```python
from build123d import *

# Parameters (mm, degrees)
SKETCH_1_R           = 2.75
SKETCH_1_R_2         = 13
EXTRUDE_1_DEPTH      = 10
EXTRUDE_1_DEPTH_BACK = 10
CUT_EXTRUDE_START    = 7.5
SKETCH_2_R           = 3.3
CUT_EXTRUDE_1_DEPTH  = 33.5
SKETCH_3_R           = 5.4
CUT_EXTRUDE_2_DEPTH  = 1.5
EXTRUDE_START        = 5.95
SKETCH_4_R           = 13
SKETCH_4_R_2         = 5
EXTRUDE_2_DEPTH      = 4
EXTRUDE_2_DEPTH_BACK = 4


with BuildPart() as part:
    # Sketch 1 → Extrude 1 (new body, two sides)
    with BuildSketch(Plane.XY) as extrude_1_sk:
        Polygon((-30, -25), (-30, 7), (-29.5, 7.5), (-17, 7.5), (-17, 17), (-16, 18), (16, 18), (17, 17), (17, 7.5), (29.5, 7.5), (30, 7), (30, -25), align=None)
        with Locations((-23, 0)):
            Circle(SKETCH_1_R, mode=Mode.SUBTRACT)
        with Locations((-23, -18)):
            Circle(SKETCH_1_R, mode=Mode.SUBTRACT)
        with Locations((23, -18)):
            Circle(SKETCH_1_R, mode=Mode.SUBTRACT)
        with Locations((23, 0)):
            Circle(SKETCH_1_R, mode=Mode.SUBTRACT)
        Circle(SKETCH_1_R_2, mode=Mode.SUBTRACT)
    extrude(amount=EXTRUDE_1_DEPTH)
    extrude(extrude_1_sk.sketch, amount=-EXTRUDE_1_DEPTH_BACK)

    # Sketch 2 → Cut-Extrude 1 (cut, through all)
    with BuildSketch(Plane(origin=(0, 0, 0), x_dir=(1, 0, 0), z_dir=(0, 1, 0)).offset(CUT_EXTRUDE_START)):
        with Locations((-23, 0)):
            Circle(SKETCH_2_R)
        with Locations((23, 0)):
            Circle(SKETCH_2_R)
    extrude(amount=-CUT_EXTRUDE_1_DEPTH, mode=Mode.SUBTRACT)

    # Sketch 3 → Cut-Extrude 2 (cut)
    with BuildSketch(Plane(origin=(0, 0, 0), x_dir=(1, 0, 0), z_dir=(0, 1, 0)).offset(CUT_EXTRUDE_START)):
        with Locations((-23, 0)):
            Circle(SKETCH_3_R)
        with Locations((23, 0)):
            Circle(SKETCH_3_R)
    extrude(amount=-CUT_EXTRUDE_2_DEPTH, mode=Mode.SUBTRACT)

    # Sketch 4 → Extrude 2 (add, two sides)
    with BuildSketch(Plane.XY.offset(EXTRUDE_START)) as extrude_2_sk:
        Circle(SKETCH_4_R)
        Circle(SKETCH_4_R_2, mode=Mode.SUBTRACT)
    extrude(amount=EXTRUDE_2_DEPTH)
    extrude(extrude_2_sk.sketch, amount=-EXTRUDE_2_DEPTH_BACK)


solid = part.part
```
Input: part model. Units: mm. Frame: model coordinates. A direction names the side the tool comes from. Round coordinates to 2 decimals unless told otherwise and drop trailing zeros. Order: outer loops, then holes, each group sorted by start corner. A loop starts at its lowest first (then second) coordinate and runs counter-clockwise, first axis right, second up. Notation, with made-up numbers: (-25.75, -9) - (9.25, -9) arc R18 ccw to (9.25, 18) - close; hole circle Ø10 at (12, 67). An arc over 180 degrees is marked (long way). One line per question, with ' | ' between items. Start each with the question number.
1) Pull-direction query (Z, two-part tool) for faces 1 (the flat face through (-30, -9, 0)), 2 (the flat face through (-6, -13, 10)), 3 (the cylindrical face through (-25.619, -9.283, 2.008)), 4 (the cylindrical face through (28.15, 6.76, -1.62)); classes: +Z half, -Z half, draft (parallel to the pull), parting line (faces both ways), or undercut.
2) Set-up query: faces 5 (the cylindrical face through (-10.316, -7.91, -3.941)), 6 (the flat face through (-23, 6, 4)), 7 (the flat face through (-17, 12, 0)), 8 (the flat face through (17, 12, 0)). Return all of +Z, -Z, +X, -X, +Y, -Y with unobstructed straight access to the full face (end or side cutting, diameter ignored); none if empty.
3) Cut plane B-B, the plane x = 23. Return the cut outline in (y, z), then the cut area to 3 significant figures.
4) Cut plane C-C, the plane z = 8.5. Return the cut outline in (x, y).
5) Ray query, probe 1 along Y at (x, z) = (23, 4.25); probe 2 along X at (y, z) = (-18, -7.5); probe 3 along Y at (x, z) = (-23, 8). Return the intervals inside material, ascending.
6) Cut plane A-A, the plane z = 0. Give the number of separate pieces and of enclosed holes in the cut face, then the cut area to 3 significant figures.
7) Contact query for flat-ended pins moving along their axis: P1, Ø8, axis at x = 4.5, y = 6, coming from the +Z side; P2, Ø5, axis at x = 23, y = -18, coming from the -Z side; P3, Ø3, axis at y = 13.5, z = -1, coming from the -X side; P4, Ø9.5, axis at x = -23, z = 0, coming from the +Y side. Output: stop coordinate, or through.
Worked out:
1) face 1: draft | face 2: +Z half | face 3: undercut | face 4: undercut
2) face 5: -Z | face 6: +Y | face 7: +Z, -Z, -X, +Y | face 8: +Z, -Z, +X, +Y
3) outline: (-25, -10) - (-20.75, -10) - (-20.75, -3.3) - (-25, -3.3) - close; (-25, 3.3) - (-20.75, 3.3) - (-20.75, 10) - (-25, 10) - close; (-15.25, -10) - (-2.75, -10) - (-2.75, -3.3) - (-15.25, -3.3) - close; (-15.25, 3.3) - (-2.75, 3.3) - (-2.75, 10) - (-15.25, 10) - close; (2.75, -10) - (7.5, -10) - (7.5, -5.4) - (6, -5.4) - (6, -3.3) - (2.75, -3.3) - close; (2.75, 3.3) - (6, 3.3) - (6, 5.4) - (7.5, 5.4) - (7.5, 10) - (2.75, 10) - close | area: 282 mm^2
4) outline: (-30, -25) - (30, -25) - (30, 7) - (29.5, 7.5) - (17, 7.5) - (17, 17) - (16, 18) - (-16, 18) - (-17, 17) - (-17, 7.5) - (-29.5, 7.5) - (-30, 7) - close; hole circle Ø5.5 at (-23, -18); hole circle Ø5.5 at (-23, 0); hole circle Ø10 at (0, 0); hole circle Ø5.5 at (23, -18); hole circle Ø5.5 at (23, 0)
5) probe 1: y = -25 to -20.75, -15.25 to -2.75, 2.75 to 6 | probe 2: x = -30 to -25.75, -20.25 to 20.25, 25.75 to 30 | probe 3: y = -25 to -20.75, -15.25 to -2.75, 2.75 to 7.5
6) separate pieces: 3 | enclosed holes: 1 | area: 1,330 mm^2
7) P1: stops at z = 9.95 | P2: passes through | P3: stops at x = -17 | P4: stops at y = 6
